```python
from build123d import *

# Parameters (mm, degrees)
BOSS_EXTRUDE1_DEPTH                                = 10
SKETCH2_W                                          = 49
SKETCH2_H                                          = 10
SKETCH3_W                                          = 1.25
SKETCH3_H                                          = 48.182761149
CBORE_FOR_M2_5_HEX_HEAD_MACHINE_SCREW1_D           = 3
CBORE_FOR_M2_5_HEX_HEAD_MACHINE_SCREW1_DEPTH       = 70.616262821
CBORE_FOR_M2_5_HEX_HEAD_MACHINE_SCREW1_CBORE_D     = 5
CBORE_FOR_M2_5_HEX_HEAD_MACHINE_SCREW1_CBORE_DEPTH = 12.433501671


with BuildPart() as part:
    # Sketch1 → Boss-Extrude1 (new body)
    with BuildSketch(Plane(origin=(0, 10, 0), x_dir=(1, 0, 0), z_dir=(0, 1, 0))):
        with BuildLine():
            Line((2.817238851, 56.91894485), (2.817238851, 48.91894485))
            ThreePointArc((2.817238851, 48.91894485), (0.317652576, 48.998970365), (-2.182761149, 48.951359059))
            Line((-2.182761149, 48.951359059), (-2.182761149, 56.951359059))
            Line((-2.182761149, 56.951359059), (-12.182761149, 56.951359059))
            Line((-12.182761149, 56.951359059), (-31.002590128, 40.494930613))
            ThreePointArc((-31.002590128, 40.494930613), (-0.248614246, -50.999394025), (31.395920468, 40.190747417))
            Line((31.395920468, 40.190747417), (12.817238851, 56.91894485))
            Line((12.817238851, 56.91894485), (2.817238851, 56.91894485))
        make_face()
    extrude(amount=-BOSS_EXTRUDE1_DEPTH)

    # Sketch2 → Cut-Revolve1 (revolve, cut)
    with BuildSketch(Plane.XY):
        with Locations((24.5, 5)):
            Rectangle(SKETCH2_W, SKETCH2_H)
    revolve(axis=Axis((0, 10, 0), (0, -1, 0)), mode=Mode.SUBTRACT)

    # Sketch3 → Ø2.5 (2.5) Diameter Hole1 (revolve, cut)
    with BuildSketch(Plane(origin=(2.817238851, 5, -52.91894485), x_dir=(0, 0, 1), z_dir=(0, 1, 0))):
        with Locations((0.625, 24.091380575)):
            Rectangle(SKETCH3_W, SKETCH3_H)
    revolve(axis=Axis((-3.532761149, 5, -52.91894485), (1, 0, 0)), mode=Mode.SUBTRACT)

    # CBORE for M2.5 Hex Head Machine Screw1
    with Locations(Plane.ZY.offset(19.616262821)):
        with Locations((-52.951359059, 5)):
            CounterBoreHole(CBORE_FOR_M2_5_HEX_HEAD_MACHINE_SCREW1_D / 2, CBORE_FOR_M2_5_HEX_HEAD_MACHINE_SCREW1_CBORE_D / 2, CBORE_FOR_M2_5_HEX_HEAD_MACHINE_SCREW1_CBORE_DEPTH, depth=CBORE_FOR_M2_5_HEX_HEAD_MACHINE_SCREW1_DEPTH)


solid = part.part
```
Verification items for the finished model (mm, model axes). A direction names the side the tool comes from. Round coordinates to 2 decimals unless told otherwise and drop trailing zeros. Write each loop counter-clockwise with the first axis right and the second up, starting at its lowest first coordinate (ties: lowest second). Pieces come first, ordered by that corner, then holes.
1. Section check A-A on x = -4.5. Enter the section's corners in (y, z).
2. Draft check along Z on faces 1 (the flat face through (-21.46, 5.07, -48.84)), 2 (the cylindrical face through (-4.648, 5.066, -51.453)), 3 (the flat face through (2.817, 5, -51)). Enter one of: +Z half, -Z half, draft (parallel to the pull), parting line (faces both ways), or undercut.
3. Access from +Z, -Z, +X, -X, +Y, -Y to the whole of each face (thin tool, end or side, straight path). Record for faces 4 (the flat face through (22.237, 5.07, -48.438)), 5 (the flat face through (-2.183, 5, -51)), 6 (the cylindrical face through (-12.105, 5.751, -50.567)).
4. Section check B-B on z = 21. Enter the section's corners in (x, y).
5. Gauge pin test, flat ends, axial feed: P1, Ø6, axis at y = 3.5, z = 15, coming from the +X side; P2, Ø4, axis at x = -34.5, y = 8, coming from the +Z side; P3, Ø3, axis at y = 6.5, z = 23, coming from the -X side. Record the tip position at first contact, or that the pin passes through.
6. Scan lines: L1, parallel to Z at x = -12.25, y = 5; L2, parallel to X at y = 3, z = 0; L3, parallel to Z at x = 11, y = 4.75. Record each from-to range of solid material in increasing order.
7. Section check C-C on x = 25. Enter the section's corners in (y, z), plus the area to 3 significant figures.
8. Section check D-D on y = 5. Enter the section's corners in (x, z).
Answer:
1. outline: (0, -56.95) - (10, -56.95) - (10, -48.79) - (0, -48.79) - close; (0, 48.79) - (10, 48.79) - (10, 50.8) - (0, 50.8) - close; hole circle Ø3 at (5, -52.95)
2. face 1: -Z half
2. face 2: undercut
2. face 3: draft
3. face 4: -Z, +X, +Y, -Y
3. face 5: -Z, +Y, -Y
3. face 6: -X
4. outline: (-46.48, 0) - (-44.27, 0) - (-44.27, 10) - (-46.48, 10) - close; (44.27, 0) - (46.48, 0) - (46.48, 10) - (44.27, 10) - close
5. P1: stops at x = 49.57
5. P2: stops at z = 39.3
5. P3: stops at x = -46.25
6. L1: z = -56.89 to -55.45, -50.45 to -47.44, 47.44 to 49.51
6. L2: x = -51 to -49, 49 to 51
6. L3: z = -56.92 to -54.43, -51.47 to -47.75, 47.75 to 49.8
7. outline: (0, -45.95) - (10, -45.95) - (10, -42.14) - (0, -42.14) - close; (0, 42.14) - (10, 42.14) - (10, 44.45) - (0, 44.45) - close
7. area: 61.2 mm2
8. outline: (-31, -40.49) - (-19.62, -50.45) - (-7.18, -50.45) - (-7.18, -51.45) - (-2.18, -51.45) - (-2.18, -48.95) arc R49 cw (long way) to (2.82, -48.92) - (2.82, -51.45) - (18.89, -51.45) - (31.4, -40.19) arc R51 ccw (long way) to start; (-13.9, -55.45) - (-12.18, -56.95) - (-2.18, -56.95) - (-2.18, -54.45) - (-7.18, -54.45) - (-7.18, -55.45) - close; (2.82, -56.92) - (12.82, -56.92) - (15.56, -54.45) - (2.82, -54.45) - close
